from build123d import *

# Parameters (mm, degrees)
AUFSATZ_LINEAR_AUSTRAGEN1_DEPTH = 100
SCHNITT_LINEAR_AUSTRAGEN1_DEPTH = 102.796365358


with BuildPart() as part:
    # Skizze1 → Aufsatz-Linear austragen1 (new body)
    with BuildSketch(Plane(origin=(0, 0, 0), x_dir=(0, 0, -1), z_dir=(1, 0, 0))):
        with BuildLine():
            Line((-3.75, 17.5), (-3.75, 13.7))
            ThreePointArc((-3.75, 13.7), (-3.603553391, 13.346446609), (-3.25, 13.2))
            Line((-3.25, 13.2), (2.95, 13.2))
            ThreePointArc((2.95, 13.2), (3.303553391, 13.053553391), (3.45, 12.7))
            Line((3.45, 12.7), (3.45, -12.7))
            ThreePointArc((3.45, -12.7), (3.303553391, -13.053553391), (2.95, -13.2))
            Line((2.95, -13.2), (-3.25, -13.2))
            ThreePointArc((-3.25, -13.2), (-3.603553391, -13.346446609), (-3.75, -13.7))
            Line((-3.75, -13.7), (-3.75, -17.5))
            Line((-3.75, -17.5), (-3.45, -17.5))
            Line((-3.45, -17.5), (-3.45, -14))
            ThreePointArc((-3.45, -14), (-3.303553391, -13.646446609), (-2.95, -13.5))
            Line((-2.95, -13.5), (3.25, -13.5))
            ThreePointArc((3.25, -13.5), (3.603553391, -13.353553391), (3.75, -13))
            Line((3.75, -13), (3.75, 13))
            ThreePointArc((3.75, 13), (3.603553391, 13.353553391), (3.25, 13.5))
            Line((3.25, 13.5), (-2.95, 13.5))
            ThreePointArc((-2.95, 13.5), (-3.303553391, 13.646446609), (-3.45, 14))
            Line((-3.45, 14), (-3.45, 17.5))
            Line((-3.45, 17.5), (-3.75, 17.5))
        make_face()
    extrude(amount=AUFSATZ_LINEAR_AUSTRAGEN1_DEPTH)

    # Skizze2 → Schnitt-Linear austragen1 (cut, through all)
    with BuildSketch(Plane(origin=(0, 0, -3.75), x_dir=(-1, 0, 0), z_dir=(0, 0, -1))):
        with BuildLine():
            Line((-95.9, 2.6), (-76.1, 2.6))
            ThreePointArc((-76.1, 2.6), (-73.5, 0), (-76.1, -2.6))
            Line((-76.1, -2.6), (-95.9, -2.6))
            ThreePointArc((-95.9, -2.6), (-98.5, 0), (-95.9, 2.6))
        make_face()
        with BuildLine():
            Line((-59.9, 2.6), (-40.1, 2.6))
            ThreePointArc((-40.1, 2.6), (-37.5, 0), (-40.1, -2.6))
            Line((-40.1, -2.6), (-59.9, -2.6))
            ThreePointArc((-59.9, -2.6), (-62.5, 0), (-59.9, 2.6))
        make_face()
        with BuildLine():
            Line((-23.9, 2.6), (-4.1, 2.6))
            ThreePointArc((-4.1, 2.6), (-1.5, 0), (-4.1, -2.6))
            Line((-4.1, -2.6), (-23.9, -2.6))
            ThreePointArc((-23.9, -2.6), (-26.5, 0), (-23.9, 2.6))
        make_face()
    extrude(amount=-SCHNITT_LINEAR_AUSTRAGEN1_DEPTH, mode=Mode.SUBTRACT)


solid = part.part
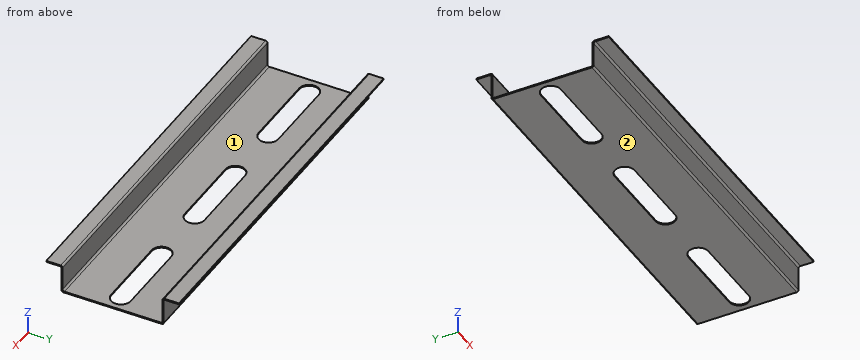
For this review, take the finished solid that the model builds, in its own axes (mm). Face numbers are marked on the shaded views. Give positions to 0.01 mm unless a question says otherwise; leave off trailing zeros. Order: outer loops, then holes, each group sorted by start corner. A loop starts at its lowest first (then second) coordinate and runs counter-clockwise, first axis right, second up. Notation, with made-up numbers: (9, 57.25) -> (13, 57.25) arc R10 cw to (13, 65.25) -> close; hole circle Ø11 at (-38.75, -9.75). An arc over 180 degrees is marked (long way). Write item = value, one per line.
1) We need section C-C, the plane y = 0. Give the boundary of the cut face in (x, z), and give its area (3 significant figures).
Findings:
outline = (0, -3.75) -> (1.5, -3.75) -> (1.5, -3.45) -> (0, -3.45) -> close; (26.5, -3.75) -> (37.5, -3.75) -> (37.5, -3.45) -> (26.5, -3.45) -> close; (62.5, -3.75) -> (73.5, -3.75) -> (73.5, -3.45) -> (62.5, -3.45) -> close; (98.5, -3.75) -> (100, -3.75) -> (100, -3.45) -> (98.5, -3.45) -> close
area = 7.50 mm^2
2) We need section D-D, the plane x = 33. Give the boundary of the cut face in (y, z).
Findings:
outline = (-17.5, 3.45) -> (-14, 3.45) arc R0.5 cw to (-13.5, 2.95) -> (-13.5, -3.25) arc R0.5 ccw to (-13, -3.75) -> (13, -3.75) arc R0.5 ccw to (13.5, -3.25) -> (13.5, 2.95) arc R0.5 cw to (14, 3.45) -> (17.5, 3.45) -> (17.5, 3.75) -> (13.7, 3.75) arc R0.5 ccw to (13.2, 3.25) -> (13.2, -2.95) arc R0.5 cw to (12.7, -3.45) -> (-12.7, -3.45) arc R0.5 cw to (-13.2, -2.95) -> (-13.2, 3.25) arc R0.5 ccw to (-13.7, 3.75) -> (-17.5, 3.75) -> close
3) To check wall thickness, follow L1, parallel to Y at x = 45.5, z = -2.25; L2, parallel to Z at x = 87.5, y = 3.5; L3, parallel to Z at x = 8.5, y = -15. State the ranges of each line that lie inside material, in increasing order. Write a range as from..to.
Findings:
L1 = -13.5..-13.2, 13.2..13.5
L2 = -3.75..-3.45
L3 = 3.45..3.75
4) We need section A-A, the plane x = 86.5. Give the boundary of the cut face in (y, z), and give its area (3 significant figures).
Findings:
outline = (-17.5, 3.45) -> (-14, 3.45) arc R0.5 cw to (-13.5, 2.95) -> (-13.5, -3.25) arc R0.5 ccw to (-13, -3.75) -> (-2.6, -3.75) -> (-2.6, -3.45) -> (-12.7, -3.45) arc R0.5 cw to (-13.2, -2.95) -> (-13.2, 3.25) arc R0.5 ccw to (-13.7, 3.75) -> (-17.5, 3.75) -> close; (2.6, -3.75) -> (13, -3.75) arc R0.5 ccw to (13.5, -3.25) -> (13.5, 2.95) arc R0.5 cw to (14, 3.45) -> (17.5, 3.45) -> (17.5, 3.75) -> (13.7, 3.75) arc R0.5 ccw to (13.2, 3.25) -> (13.2, -2.95) arc R0.5 cw to (12.7, -3.45) -> (2.6, -3.45) -> close
area = 13.3 mm^2
5) Draft analysis for pull direction Y (two halves, no side actions). For the marked faces 1 and 2, state which applies: pulls with the +Y half, pulls with the -Y half, needs draft (parallel to the pull), parting line crosses it, or undercut.
Findings:
face_1 = undercut
face_2 = needs draft
6) We need section B-B, the plane z = -0.5. Give the boundary of the cut face in (x, y).
Findings:
outline = (0, -13.5) -> (100, -13.5) -> (100, -13.2) -> (0, -13.2) -> close; (0, 13.2) -> (100, 13.2) -> (100, 13.5) -> (0, 13.5) -> close
7) Insertion check: pin 1 (12.5 mm diameter, centred on x = 50.5, y = -5.5, fed in from +Z); pin 2 (1.8 mm diameter, centred on x = 47, y = 15.5, fed in from -Z); pin 3 (3 mm diameter, centred on x = 38, z = 0.5, fed in from -Y). Each pin has a flat end and moves straight along its axis. Give the tip position at first contact, or say it passes through.
Findings:
pin_1 = -3.45
pin_2 = 3.45
pin_3 = -13.5
